Geometry: see drawing. Coordinates: mm, zero at the bounding-box minimum. Coordinates: 2 decimals unless noted, no trailing zeros. Order: outer loops, then holes, each group sorted by start corner. A loop starts at its lowest first (then second) coordinate and runs counter-clockwise, first axis right, second up.
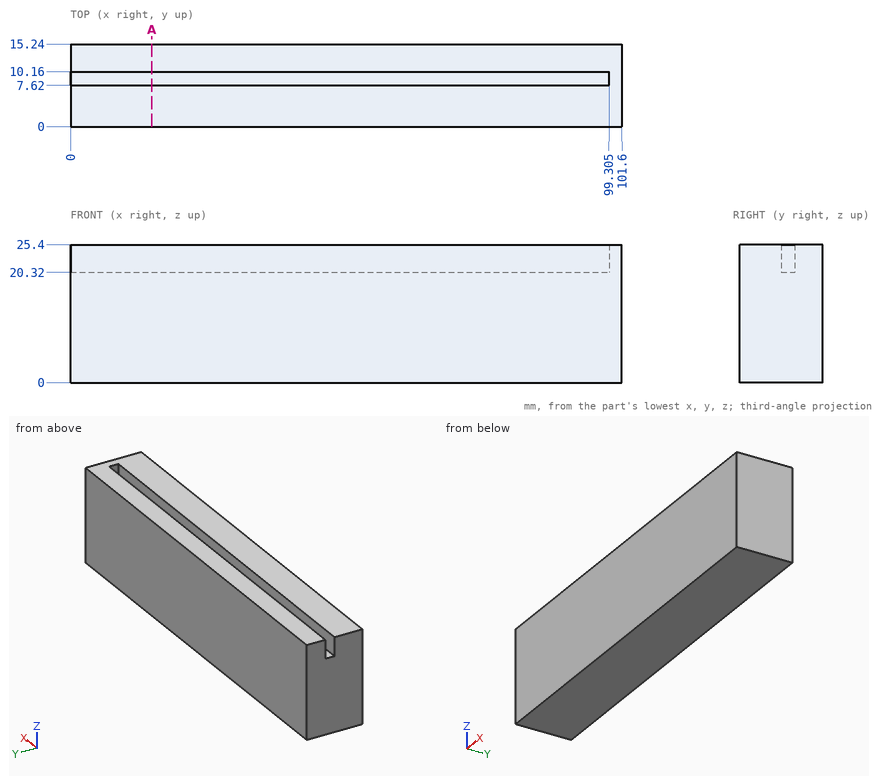
Item 1: Pin query (flat end, axial travel): pin 1 Ø1.3 at (x, y) = (48, 8.5) entering from +Z. Return the tip coordinate at first contact, or that it passes through.
Response values:
pin 1: stops at z = 20.32
Item 2: Cut plane A-A on x = 15. Return loops of the section in (y, z), then the cut area to 3 significant figures.
Response values:
outline: (0, 0) - (15.24, 0) - (15.24, 25.4) - (10.16, 25.4) - (10.16, 20.32) - (7.62, 20.32) - (7.62, 25.4) - (0, 25.4) - close
area: 374 mm2
Item 3: Ray query, probe 1 along Y at (x, z) = (92, 21.75); probe 2 along Z at (x, y) = (28, 9.25). Return the intervals inside material, ascending.
Response values:
probe 1: y = 0 to 7.62, 10.16 to 15.24
probe 2: z = 0 to 20.32
